Source: three-view drawing plus pictorial views. Frame: mm from the lowest corner of the part. A direction names the side the tool comes from. Coordinates: 2 decimals unless noted, no trailing zeros. Loops run counter-clockwise (first coordinate to the right, second up) from the corner with the lowest first, then second, coordinate; pieces in that order, holes last. Notation, with made-up numbers: (-29.5, -29.75) - (-8.5, -29.75) arc R18 ccw to (-8.5, -17.75) - close; hole circle Ø7 at (-31.75, 70.25). An arc over 180 degrees is marked (long way). Return JSON: item names as keys, results as strings.
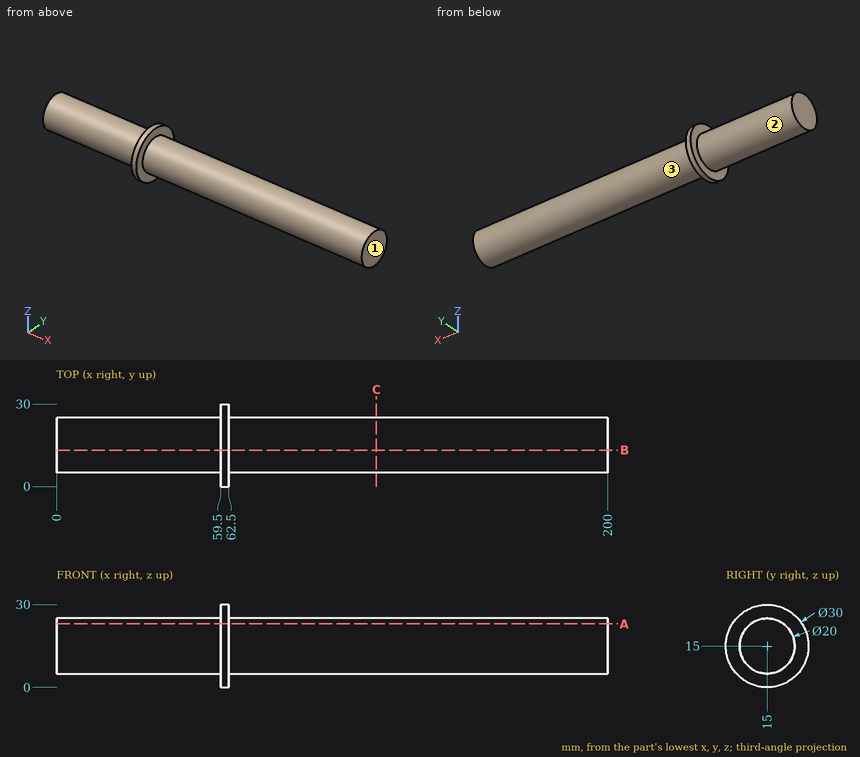
Item 1: First-contact query: pin 1 Ø1 at (x, z) = (27.5, 26.5) entering from +Y; pin 2 Ø1.5 at (x, z) = (149, 15) entering from -Y; pin 3 Ø3 at (x, z) = (65, 18) entering from +Y; pin 4 Ø5 at (x, y) = (176.5, 12) entering from -Z. Flat tips, straight axial feed; report the tip coordinate or a pass-through.
Worked out:
{"pin 1": "through", "pin 2": "y = 5", "pin 3": "y = 24.89", "pin 4": "z = 5.01"}
Item 2: Section query A-A, the plane z = 23. Return loops of the section in (x, y), and give its area (3 significant figures).
Worked out:
{"outline": "(0, 9) - (59.5, 9) - (59.5, 2.31) - (62.5, 2.31) - (62.5, 9) - (200, 9) - (200, 21) - (62.5, 21) - (62.5, 27.69) - (59.5, 27.69) - (59.5, 21) - (0, 21) - close", "area": "2,440 mm^2"}
Item 3: Section query B-B, the plane y = 13.25. Return loops of the section in (x, z).
Worked out:
{"outline": "(0, 5.15) - (59.5, 5.15) - (59.5, 0.1) - (62.5, 0.1) - (62.5, 5.15) - (200, 5.15) - (200, 24.85) - (62.5, 24.85) - (62.5, 29.9) - (59.5, 29.9) - (59.5, 24.85) - (0, 24.85) - close"}
Item 4: Ray query, probe 1 along X at (y, z) = (4.25, 4.75); probe 2 along Y at (x, z) = (88.5, 6.5); probe 3 along Y at (x, z) = (12.5, 18.5). Return the intervals inside material, ascending. Write a range as from..to.
Worked out:
{"probe 1": "59.5..62.5", "probe 2": "9.73..20.27", "probe 3": "5.63..24.37"}
Item 5: Reachability of the marked faces 1, 2 and 3 from +Z, -Z, +X, -X, +Y, -Y: full face, straight path, thin tool, end or side. Return the list, or none.
Worked out:
{"face 1": "+Z, -Z, +X, +Y, -Y", "face 2": "-X", "face 3": "+X"}
Item 6: Section query C-C, the plane x = 116. Return loops of the section in (y, z).
Worked out:
{"outline": "circle Ø20 at (15, 15)"}
